Part print with two shaded views. Sizes in mm from the minimum x, y, z corner. A direction names the side the tool comes from. Round coordinates to 2 decimals unless told otherwise and drop trailing zeros. Loops run counter-clockwise (first coordinate to the right, second up) from the corner with the lowest first, then second, coordinate; pieces in that order, holes last.
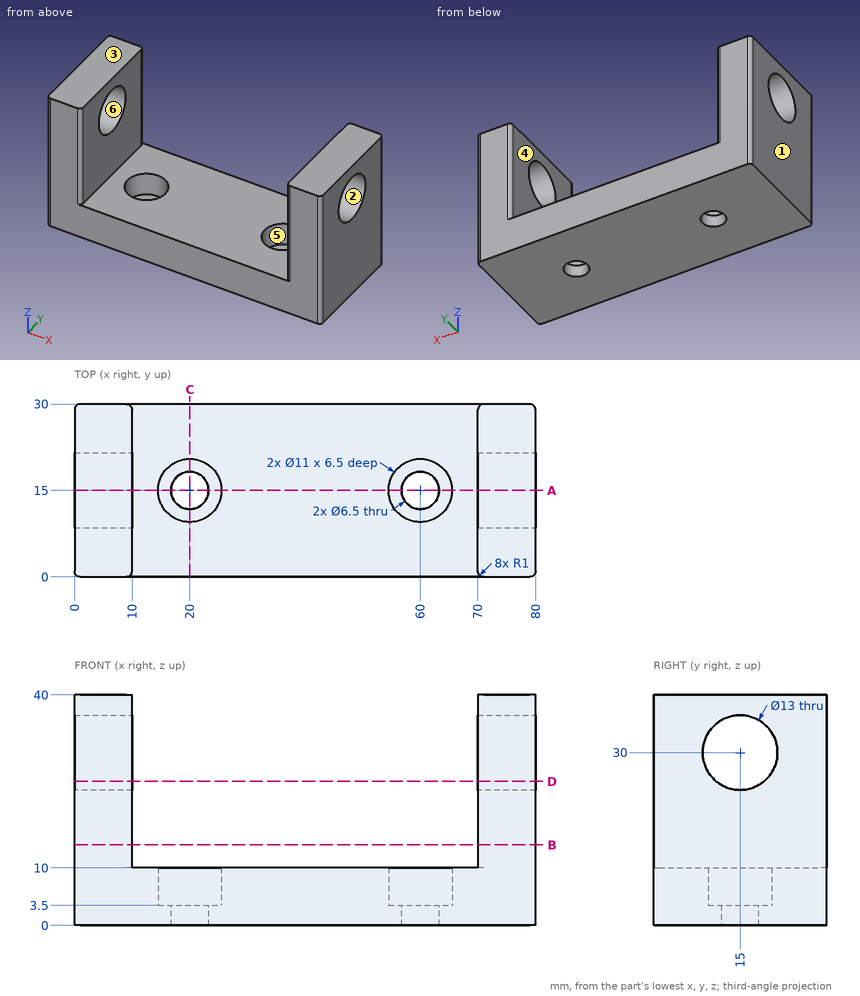
Item 1: Cut at C-C (x = 20). List the corners of the cut face in (y, z), plus the area to 3 significant figures.
Verdict:
outline: (0, 0) - (11.75, 0) - (11.75, 3.5) - (9.5, 3.5) - (9.5, 10) - (0, 10) - close; (18.25, 0) - (30, 0) - (30, 10) - (20.5, 10) - (20.5, 3.5) - (18.25, 3.5) - close
area: 206 mm2
Item 2: Cut at A-A (y = 15). State how many separate pieces and enclosed holes the cut face has, plus the area to 4 significant figures.
Verdict:
separate pieces: 5
enclosed holes: 0
area: 951.5 mm2
Item 3: Mould opens along Z. For the marked faces 1, 2 and 3 say: released by +Z, released by -Z, zero draft, split by the parting line, or undercut.
Verdict:
face 1: zero draft
face 2: undercut
face 3: released by +Z
Item 4: Flat gauge pins, fed straight in: P1, Ø10, axis at x = 61.5, y = 13, coming from the +Z side; P2, Ø8, axis at y = 15, z = 30, coming from the +X side; P3, Ø3.5, axis at x = 62.5, y = 13, coming from the +Z side. Where does each tip first touch, or does it go through?
Verdict:
P1: stops at z = 10
P2: passes through
P3: stops at z = 3.5
Item 5: 3-axis set-ups, long thin cutter, end or side, ignore diameter. For the marked faces 4, 5 and 6: which of +Z, -Z, +X, -X, +Y, -Y reach the whole face in a straight line?
Verdict:
face 4: +Z, +Y, -Y
face 5: +Z
face 6: +X, -X
Item 6: Wall check: L1, parallel to X at y = 15, z = 1.75; L2, parallel to X at y = 15, z = 5; L3, parallel to X at y = 10.75, z = 35. Give the ranges that are in metal, low to high.
Verdict:
L1: x = 0 to 16.75, 23.25 to 56.75, 63.25 to 80
L2: x = 0 to 14.5, 25.5 to 54.5, 65.5 to 80
L3: x = 0 to 10, 70 to 80
Item 7: Cut at D-D (z = 25). List the corners of the cut face in (x, y), plus the area to 3 significant figures.
Verdict:
outline: (0, 1) arc R1 ccw to (1, 0) - (9, 0) arc R1 ccw to (10, 1) - (10, 10.85) - (0, 10.85) - close; (0, 19.15) - (10, 19.15) - (10, 29) arc R1 ccw to (9, 30) - (1, 30) arc R1 ccw to (0, 29) - close; (70, 1) arc R1 ccw to (71, 0) - (79, 0) arc R1 ccw to (80, 1) - (80, 10.85) - (70, 10.85) - close; (70, 19.15) - (80, 19.15) - (80, 29) arc R1 ccw to (79, 30) - (71, 30) arc R1 ccw to (70, 29) - close
area: 432 mm2
Item 8: Cut at B-B (z = 14). List the corners of the cut face in (x, y), plus the area to 3 significant figures.
Verdict:
outline: (0, 1) arc R1 ccw to (1, 0) - (9, 0) arc R1 ccw to (10, 1) - (10, 29) arc R1 ccw to (9, 30) - (1, 30) arc R1 ccw to (0, 29) - close; (70, 1) arc R1 ccw to (71, 0) - (79, 0) arc R1 ccw to (80, 1) - (80, 29) arc R1 ccw to (79, 30) - (71, 30) arc R1 ccw to (70, 29) - close
area: 598 mm2
